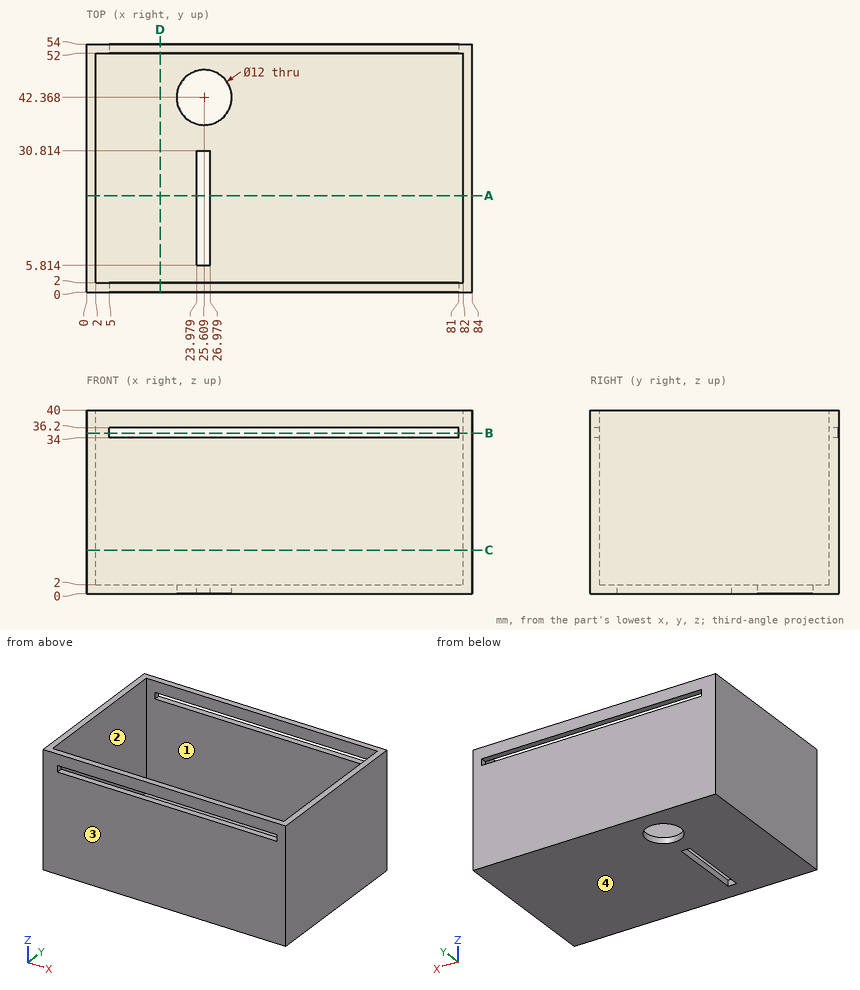
Design review of the part shown in the three views and the two pictorial views. Dimensions are in mm from the part's minimum x, y and z. Give positions to 0.01 mm unless a question says otherwise; leave off trailing zeros. Loops run counter-clockwise (first coordinate to the right, second up) from the corner with the lowest first, then second, coordinate; pieces in that order, holes last. Notation, with made-up numbers: (-11.5, 17.25) - (29.5, 17.25) arc R20 ccw to (29.5, 47.25) - close; hole circle Ø4 at (60, 74.25). An arc over 180 degrees is marked (long way). Answer as a JSON object with one key per item and string values.
Q1. Add section D-D on x = 16. State the section outline as (y, z) points, plus the area to 3 significant figures.
Worked out:
{"outline": "(0, 0) - (54, 0) - (54, 34) - (52, 34) - (52, 2) - (2, 2) - (2, 34) - (0, 34) - close; (0, 36.2) - (2, 36.2) - (2, 40) - (0, 40) - close; (52, 36.2) - (54, 36.2) - (54, 40) - (52, 40) - close", "area": "251 mm^2"}
Q2. Add section C-C on z = 9.5. State the section outline as (x, y) points, plus the area to 3 significant figures.
Worked out:
{"outline": "(0, 0) - (84, 0) - (84, 54) - (0, 54) - close; hole (2, 2) - (82, 2) - (82, 52) - (2, 52) - close", "area": "536 mm^2"}
Q3. To check wall thickness, follow line 1 along Y through (x, z) = (43, 4.5); line 2 along X through (y, z) = (11, 11.5); line 3 along Z through (x, y) = (33, 33). State the ranges of each line that lie inside material, in increasing order.
Worked out:
{"line 1": "y = 0 to 2, 52 to 54", "line 2": "x = 0 to 2, 82 to 84", "line 3": "z = 0 to 2"}
Q4. Insertion check: pin 1 (12 mm diameter, centred on x = 64.5, y = 28.5, fed in from +Z); pin 2 (12 mm diameter, centred on x = 45.5, z = 30, fed in from -Y). Each pin has a flat end and moves straight along its axis. Give the tip position at first contact, or say it passes through.
Worked out:
{"pin 1": "stops at z = 2", "pin 2": "stops at y = 0"}
Q5. Add section B-B on z = 35. State the section outline as (x, y) points, plus the area to 3 significant figures.
Worked out:
{"outline": "(0, 0) - (5, 0) - (5, 2) - (2, 2) - (2, 52) - (5, 52) - (5, 54) - (0, 54) - close; (81, 0) - (84, 0) - (84, 54) - (81, 54) - (81, 52) - (82, 52) - (82, 2) - (81, 2) - close", "area": "232 mm^2"}
Q6. Add section A-A on y = 21. State the section outline as (x, z) points, plus the area to 3 significant figures.
Worked out:
{"outline": "(0, 0) - (23.98, 0) - (23.98, 2) - (2, 2) - (2, 40) - (0, 40) - close; (26.98, 0) - (84, 0) - (84, 40) - (82, 40) - (82, 2) - (26.98, 2) - close", "area": "314 mm^2"}
Q7. Mouldability with a two-part tool opening along Y and no side actions: class the marked faces 1, 2, 3 and 4 as +Y half, -Y half, draft (parallel to the pull), parting line (faces both ways), or undercut.
Worked out:
{"face 1": "undercut", "face 2": "undercut", "face 3": "-Y half", "face 4": "draft"}
